The drawing under review shows one solid part. Ordinate dimensions are in mm from its lowest x, y, z. A direction names the side the tool comes from. Round coordinates to 2 decimals unless told otherwise and drop trailing zeros. Write each loop counter-clockwise with the first axis right and the second up, starting at its lowest first coordinate (ties: lowest second). Pieces come first, ordered by that corner, then holes. Notation, with made-up numbers: (34, 65.25) -> (78, 65.25) arc R21 cw to (78, 90.25) -> close; hole circle Ø6 at (59.25, 39.25). An arc over 180 degrees is marked (long way). Use CSV: the item, a comma, the result in double quotes. Start each with the question number.
1) Take a section at A-A, the plane y = 19.05. Give the boundary of the cut face in (x, z).
2) Take a section at C-C, the plane x = 19.05. Give the boundary of the cut face in (y, z), then the cut area to 3 significant figures.
3) For pin 1 Ø1.5 at (y, z) = (20.5, 2) entering from -X; pin 2 Ø3 at (x, z) = (32.5, 5.5) entering from +Y (1 decimal); pin 3 Ø3 at (y, z) = (19.5, 3) entering from +X; pin 4 Ø1 at (y, z) = (25, 3.5) entering from +X, all flat-tipped, find the tip position at first contact; note any pin that passes through.
4) Wall thickness on probe 1 along Y at (x, z) = (19.05, 6.6); probe 2 along Z at (x, y) = (4, 17); probe 3 along Y at (x, z) = (19.05, 6.95): over which ranges is each line inside the solid? List them lowest first. Write a range as [from, to].
5) Mouldability with a two-part tool opening along X and no side actions: class the marked faces 3, 4 and 5 as released by +X, released by -X, zero draft, split by the parting line, or undercut.
6) Take a section at D-D, the plane z = 1.5. Give the boundary of the cut face in (x, y), then the cut area to 3 significant figures.
7) Machinability: for the marked faces 1 and 2, which of the approach directions +Z, -Z, +X, -X, +Y, -Y give a long, thin tool a straight path to every point of the face, cutting with its end or side? Answer none if there is none.
8) Take a section at B-B, the plane z = 5.5. Give the boundary of the cut face in (x, y), then the cut area to 3 significant figures.
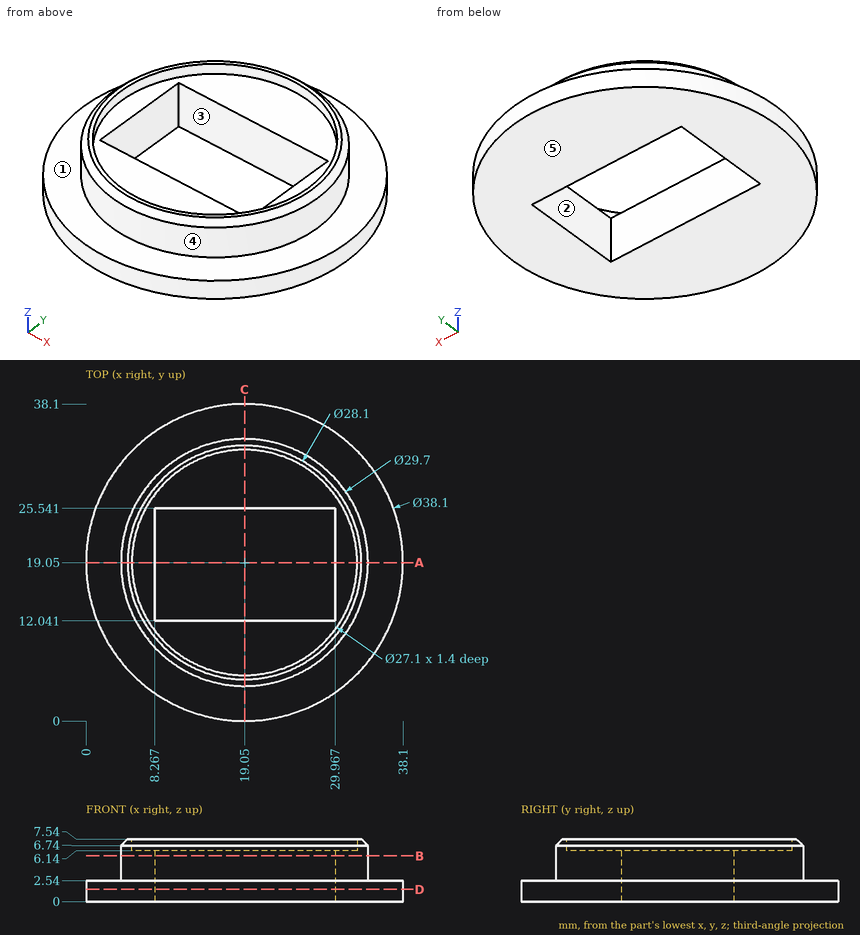
Values found:
1,outline,"(0, 0) -> (8.27, 0) -> (8.27, 6.14) -> (5.5, 6.14) -> (5.5, 7.54) -> (5, 7.54) -> (4.2, 6.74) -> (4.2, 2.54) -> (0, 2.54) -> close; (29.97, 0) -> (38.1, 0) -> (38.1, 2.54) -> (33.9, 2.54) -> (33.9, 6.74) -> (33.1, 7.54) -> (32.6, 7.54) -> (32.6, 6.14) -> (29.97, 6.14) -> close"
2,outline,"(0, 0) -> (12.04, 0) -> (12.04, 6.14) -> (5.5, 6.14) -> (5.5, 7.54) -> (5, 7.54) -> (4.2, 6.74) -> (4.2, 2.54) -> (0, 2.54) -> close; (25.54, 0) -> (38.1, 0) -> (38.1, 2.54) -> (33.9, 2.54) -> (33.9, 6.74) -> (33.1, 7.54) -> (32.6, 7.54) -> (32.6, 6.14) -> (25.54, 6.14) -> close"
2,area,"124 mm²"
3,pin 1,"x = 0.01"
3,pin 2,"y = 27.9"
3,pin 3,"x = 38.1"
3,pin 4,"x = 32.86"
4,probe 1,"[4.2, 5.5], [32.6, 33.9]"
4,probe 2,"[0, 2.54]"
4,probe 3,"[4.41, 5.5], [32.6, 33.69]"
5,face 3,"undercut"
5,face 4,"split by the parting line"
5,face 5,"zero draft"
6,outline,"circle Ø38.1 at (19.05, 19.05); hole (8.27, 12.04) -> (29.97, 12.04) -> (29.97, 25.54) -> (8.27, 25.54) -> close"
6,area,"847 mm²"
7,face 1,"+Z"
7,face 2,"+Z, -Z"
8,outline,"circle Ø29.7 at (19.05, 19.05); hole (8.27, 12.04) -> (29.97, 12.04) -> (29.97, 25.54) -> (8.27, 25.54) -> close"
8,area,"400 mm²"
